Autodesk Inventor part; units mm, degrees
ref_plane "YZ Plane" through (0, 0, 0) normal (1, 0, 0) x (0, 1, 0)
ref_plane "XZ Plane" through (0, 0, 0) normal (0, 1, 0) x (-1, 0, 0)
ref_plane "XY Plane" through (0, 0, 0) normal (0, 0, 1) x (1, 0, 0)
sketch "Sketch1" plane through (0, 0, 0) normal (0, 0, 1) x (1, 0, 0)
  line L0 (0, 0) -> (-29, 0)
  line L1 (-29, 0) -> (-29, 4)
  line L2 (-29, 4) -> (-4, 4)
  line L3 (-4, 4) -> (-4, 18)
  line L4 (-4, 18) -> (0, 18)
  line L5 (0, 18) -> (0, 0)
  dimension "d0" = 4
  dimension "d1" = 4
  dimension "d2" = 29
  dimension "d3" = 18
extrude "Extrusion1" add sketch "Sketch1" along normal blind 80
sketch "Sketch2" plane through (0, 0, 0) normal (1, 0, 0) x (0, 0, -1)
  line L0 (0, 4) -> (-80, 4)
  line L1 (-51, 18) -> (-29, 18)
  line L2 (-29, 18) -> (-29, 4)
  line L3 (-29, 4) -> (-51, 4)
  line L4 (-51, 4) -> (-51, 18)
  line L5 (0, 18) -> (-80, 18)
  point P0 (0, 0)
  point P1 (-40, 18)
  point P2 (-40, 4)
  point P3 (-51, 4)
  dimension "d6" = 22
extrude "Extrusion2" cut sketch "Sketch2" against normal through all
sketch "Sketch3" plane through (0, 0, 0) normal (1, 0, 0) x (0, 0, -1)
  line L0 (0, 0) -> (-80, 0)
  line L1 (-80, 0) -> (-80, 18)
  line L2 (0, 0) -> (0, 18)
  point P0 (-70, 9)
  point P1 (-10, 9)
  dimension "d9" = 9
  dimension "d10" = 10
  dimension "d11" = 10
hole "Hole1" at (0, 9, 70) at (0, 9, 10) direction (-1, 0, 0) diameter 5.5 end through all
sketch "Sketch4" plane through (-29, 0, 0) normal (0, -1, 0) x (1, 0, 0)
  line L0 (29, 0) -> (29, 80)
  line L1 (0, 0) -> (29, 0)
  point P0 (20, 60)
  point P1 (20, 20)
  dimension "d19" = 9
  dimension "d20" = 20
  dimension "d21" = 20
hole "Hole2" at (-9, 0, 60) at (-9, 0, 20) direction (0, 1, 0) diameter 5.5 end through all
sketch "Sketch5" plane through (-29, 4, 0) normal (0, 1, 0) x (1, 0, 0)
  line L0 (0, 0) -> (0, -80)
  line L1 (0, -52.8652) -> (19, -80)
  line L2 (25, -80) -> (0, -80)
  line L3 (25, 0) -> (0, 0)
  line L4 (19, 0) -> (0, -27.1348)
  line L5 (25, -29) -> (29, -29)
  line L6 (29, -51) -> (25, -51)
  line L7 (29, -51) -> (29, -80)
  line L8 (29, 0) -> (29, -29)
  dimension "d29" = 10
  dimension "d30" = 10
  dimension "d31" = 55
  dimension "d32" = 55
extrude "Extrusion3" cut sketch "Sketch5" against normal through all
sketch "Sketch6" plane through (-4, 4, 51) normal (0, 1, 0) x (1, 0, 0)
  line L0 (4, 22) -> (4, 0)
  line L1 (-25, 23.8652) -> (-25, -1.8652)
  point P0 (4, 51)
  point P1 (-4, 11)
  point P2 (-17, 11)
  point P3 (-25, 11)
  dimension "d35" = 8
  dimension "d36" = 8
hole "Hole3" at (-8, 4, 40) at (-21, 4, 40) direction (0, -1, 0) diameter 4.5 end through all
sketch "Sketch7" plane through (-29, 0, 27.1348) normal (-1, 0, 0) x (0, 0, 1)
  line L0 (0, 4) -> (0, 0)
  line L1 (0, 0) -> (25.7304, 0)
  line L2 (25.7304, 0) -> (25.7304, 4)
  line L3 (0, 4) -> (25.7304, 4)
  line L4 (0, 0) -> (25.7304, 0)
  line L5 (25.7304, 0) -> (25.7304, 18)
  line L6 (25.7304, 18) -> (0, 18)
  line L7 (0, 18) -> (0, 0)
  line L8 (25.7304, 0) -> (25.7304, 4)
  line L9 (-27.1348, 18) -> (1.8652, 18)
  point P0 (-27.1348, 0)
extrude "Extrusion4" add sketch "Sketch7" along normal blind 4
sketch "Sketch8" plane through (-33, 0, 27.1348) normal (-1, 0, 0) x (0, 0, 1)
  line L0 (25.7304, 18) -> (0, 18)
  line L1 (-27.1348, 4) -> (0, 4)
  point P0 (-27.1348, 0)
  point P1 (12.8652, 14)
  point P2 (12.8652, 18)
  dimension "d46" = 10
hole "Hole4" at (-33, 14, 40) direction (1, 0, 0) diameter 5.5 end through all
chamfer "Chamfer1" distance 5 angle 45 2 edges at (-31, 18, 27.1348) (-31, 18, 52.8652)
equation "\"d30\" = d29"
equation "\"d32\" = d31"
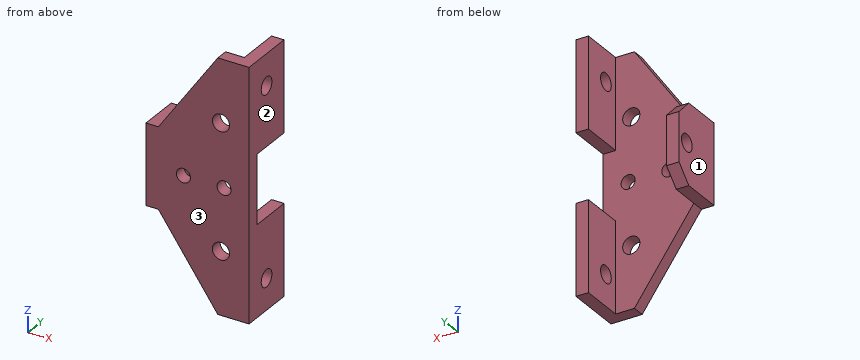
CAD build for the part. Positions are in the model's coordinates, mm. Face numbers are marked on the shaded views. Round coordinates to 2 decimals unless told otherwise and drop trailing zeros. Write each loop counter-clockwise with the first axis right and the second up, starting at its lowest first coordinate (ties: lowest second). Pieces come first, ordered by that corner, then holes. Notation, with made-up numbers: M 40,-13.75 L 62,-13.75 A17 cw 62,-4.75 Z; hole C 3,10.25 d4. An arc over 180 degrees is marked long. One line per question, with ' | ' between items.
1. Probe L1, parallel to X at y = 3.2, z = 40; L2, parallel to X at y = 11, z = 34; L3, parallel to Z at x = -9, y = 1.85. List the from-to ranges inside material, lowest first. Write a range as from..to.
Working result:
L1: -33..-23.25, -18.75..-10.25, -5.75..0 | L2: -33..-29 | L3: 0..17.25, 22.75..37.98, 42.02..57.25, 62.75..80
2. Cut at D-D on y = 14. Write the cut outline in (x, z).
Working result:
outline: M -33,28.13 L -29,28.13 L -29,37.25 L -33,37.25 Z; M -33,42.75 L -29,42.75 L -29,51.87 L -33,51.87 Z; M -4,0 L 0,0 L 0,29 L -4,29 Z; M -4,51 L 0,51 L 0,80 L -4,80 Z
3. Mould opens along X. For the marked faces 1, 2 and 3 say: pulls with the +X half, pulls with the -X half, needs draft (parallel to the pull), parting line crosses it, or undercut.
Working result:
face 1: pulls with the -X half | face 2: pulls with the +X half | face 3: needs draft
4. Cut at C-C on z = 18.5. Write the cut outline in (x, y).
Working result:
outline: M -22.95,0 L -11.3,0 L -11.3,4 L -22.95,4 Z; M -6.7,0 L 0,0 L 0,18 L -4,18 L -4,4 L -6.7,4 Z
5. Cut at A-A on y = 9. Write the cut outline in (x, z).
Working result:
outline: M -33,27.13 L -29,27.13 L -29,52.87 L -33,52.87 Z; M -4,0 L 0,0 L 0,7.25 L -4,7.25 Z; M -4,12.75 L 0,12.75 L 0,29 L -4,29 Z; M -4,51 L 0,51 L 0,67.25 L -4,67.25 Z; M -4,72.75 L 0,72.75 L 0,80 L -4,80 Z
6. Cut at B-B on x = -21. Write the cut outline in (y, z), and give its area (3 significant figures).
Working result:
outline: M 0,15.71 L 4,15.71 L 4,37.75 L 0,37.75 Z; M 0,42.25 L 4,42.25 L 4,64.29 L 0,64.29 Z | area: 176 mm2
7. Pin check, flat tips, straight feed: pin 1 Ø2 at (y, z) = (6.5, 67.5) entering from -X; pin 2 Ø6 at (x, z) = (-7.5, 31) entering from +Y; pin 3 Ø3 at (x, y) = (-31, 6.5) entering from -Z. Stop position of each tip, or through.
Working result:
pin 1: x = -4 | pin 2: y = 4 | pin 3: z = 27.13
